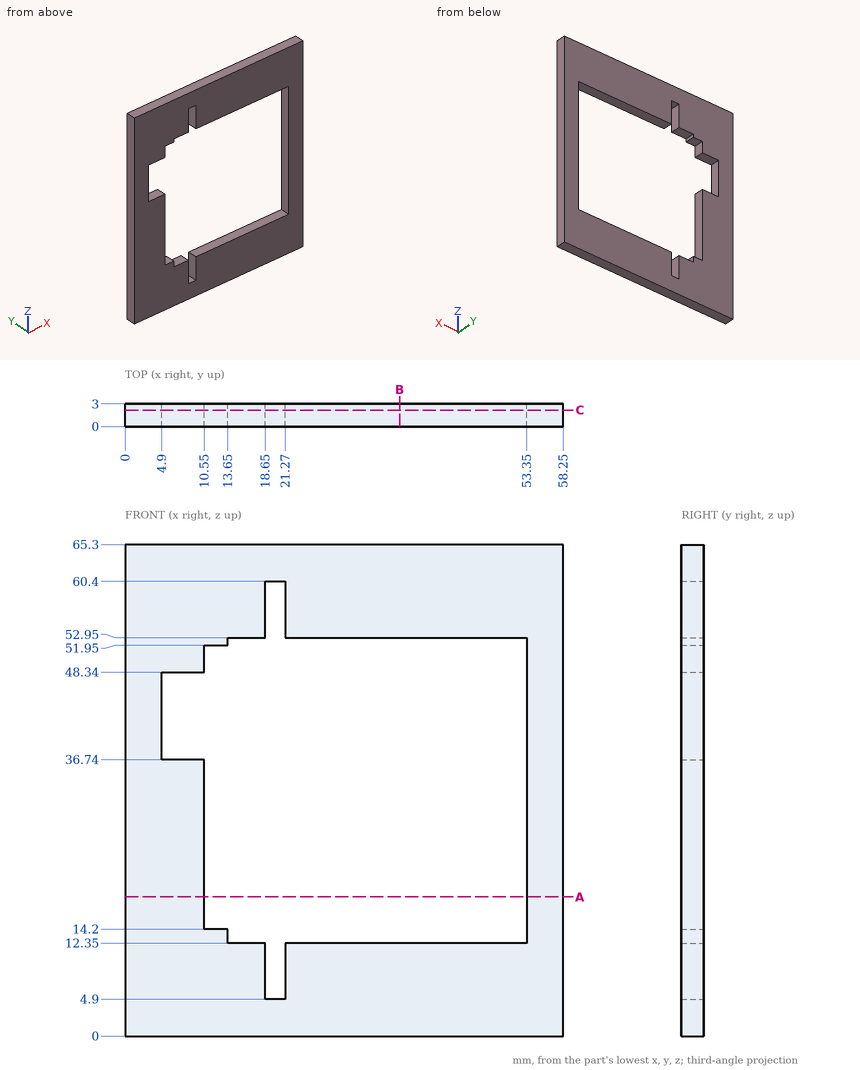
Verification items for this drawing (mm, ordinates from the low corner). Give positions to 0.01 mm unless a question says otherwise; leave off trailing zeros. Write each loop counter-clockwise with the first axis right and the second up, starting at its lowest first coordinate (ties: lowest second). Pieces come first, ordered by that corner, then holes. Notation, with made-up numbers: (-7.75, 0) - (29.25, 0) arc R28 cw to (29.25, 30) - close; hole circle Ø5 at (75, 65). An arc over 180 degrees is marked (long way). Answer as CSV lines item,"result". Start each with the question number.
1. Sectioned sample at C-C (y = 2.2). Record the boundary of the cut face in (x, z), then the cut area to 3 significant figures.
2. Sectioned sample at B-B (x = 36.5). Record the boundary of the cut face in (y, z).
3. Sectioned sample at A-A (z = 18.5). Record the boundary of the cut face in (x, y), then the cut area to 4 significant figures.
4. Thickness scan on line 1 (Z direction, x = 37, y = 1.7); line 2 (X direction, y = 1.45, z = 34); line 3 (Z direction, x = 5.5, y = 2.5). Record the ranges inside material, lowest first.
Derived:
1,outline,"(0, 0) - (58.25, 0) - (58.25, 65.3) - (0, 65.3) - close; hole (4.9, 36.74) - (10.55, 36.74) - (10.55, 14.2) - (13.65, 14.2) - (13.65, 12.35) - (18.65, 12.35) - (18.65, 4.9) - (21.27, 4.9) - (21.27, 12.35) - (53.35, 12.35) - (53.35, 52.95) - (21.27, 52.95) - (21.27, 60.4) - (18.65, 60.4) - (18.65, 52.95) - (13.65, 52.95) - (13.65, 51.95) - (10.55, 51.95) - (10.55, 48.34) - (4.9, 48.34) - close"
1,area,"1,970 mm²"
2,outline,"(0, 0) - (3, 0) - (3, 12.35) - (0, 12.35) - close; (0, 52.95) - (3, 52.95) - (3, 65.3) - (0, 65.3) - close"
3,outline,"(0, 0) - (10.55, 0) - (10.55, 3) - (0, 3) - close; (53.35, 0) - (58.25, 0) - (58.25, 3) - (53.35, 3) - close"
3,area,"46.35 mm²"
4,line 1,"0 to 12.35, 52.95 to 65.3"
4,line 2,"0 to 10.55, 53.35 to 58.25"
4,line 3,"0 to 36.74, 48.34 to 65.3"
